Can you work these out from the model? Positions are in its coordinate system, mm. Face numbers are marked on the shaded views. A direction names the side the tool comes from. Coordinates: 2 decimals unless noted, no trailing zeros. Loops run counter-clockwise (first coordinate to the right, second up) from the corner with the lowest first, then second, coordinate; pieces in that order, holes last.
```python
from build123d import *

# Parameters (mm, degrees)
SALIENTE_EXTRUIR1_DEPTH      = 18.75
SALIENTE_EXTRUIR1_DEPTH_BACK = 18.75
CROQUIS1_R                   = 2.45
CROQUIS3_R                   = 1
CORTAR_EXTRUIR1_DEPTH        = 8


with BuildPart() as part:
    # Croquis1 → Saliente-Extruir1 (new, two sides: drawn at the far end of the back side and taken through both)
    with BuildSketch(Plane.XY.offset(-SALIENTE_EXTRUIR1_DEPTH_BACK)):
        Circle(CROQUIS1_R)
    extrude(amount=SALIENTE_EXTRUIR1_DEPTH + SALIENTE_EXTRUIR1_DEPTH_BACK)

    # Croquis3 → Cortar-Extruir1 (cut)
    with BuildSketch(Plane.XY.offset(18.75)):
        Circle(CROQUIS3_R)
        with BuildLine():
            Line((-1.71464282, 1.75), (1.71464282, 1.75))
            ThreePointArc((1.71464282, 1.75), (0, 2.45), (-1.71464282, 1.75))
        make_face()
        with BuildLine():
            Line((-1.71464282, -1.75), (1.71464282, -1.75))
            ThreePointArc((1.71464282, -1.75), (0, -2.45), (-1.71464282, -1.75))
        make_face()
    cortar_extruir1 = extrude(amount=-CORTAR_EXTRUIR1_DEPTH, mode=Mode.SUBTRACT)

    # Simetría1: Cortar-Extruir1 across plane
    add(cortar_extruir1.mirror(Plane.XY), mode=Mode.SUBTRACT)


solid = part.part
```
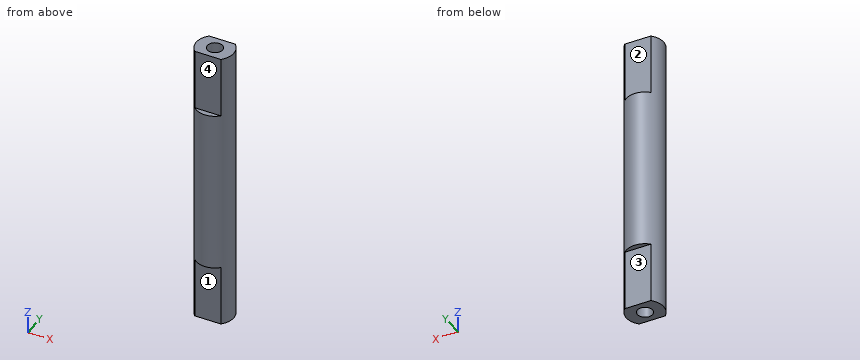
Item 1: On a 3-axis mill with a long thin cutter (end or side, diameter ignored), from which of +Z, -Z, +X, -X, +Y, -Y can I reach the whole of each face in a straight line? I mean the marked faces 1, 2, 3 and 4. Say none if no direction works.
Results are:
face 1: -Z, +X, -X, -Y
face 2: +Z, +X, -X, +Y
face 3: -Z, +X, -X, +Y
face 4: +Z, +X, -X, -Y
Item 2: Suppose I cut it at D-D, the plane z = -2.5. Please give me the cut outline in (x, y), plus the area to 3 significant figures.
Results are:
outline: circle Ø4.9 at (0, 0)
area: 18.9 mm2
Item 3: Suppose I cut it at B-B, the plane x = 0. Please give me the cut outline in (y, z).
Results are:
outline: (-2.45, -10.75) - (-1.75, -10.75) - (-1.75, -18.75) - (-1, -18.75) - (-1, -10.75) - (1, -10.75) - (1, -18.75) - (1.75, -18.75) - (1.75, -10.75) - (2.45, -10.75) - (2.45, 10.75) - (1.75, 10.75) - (1.75, 18.75) - (1, 18.75) - (1, 10.75) - (-1, 10.75) - (-1, 18.75) - (-1.75, 18.75) - (-1.75, 10.75) - (-2.45, 10.75) - close
Item 4: Suppose I cut it at A-A, the plane z = 13.5. Please give me the cut outline in (x, y), plus the area to 3 significant figures.
Results are:
outline: (-1.71, -1.75) - (1.71, -1.75) arc R2.45 ccw to (1.71, 1.75) - (-1.71, 1.75) arc R2.45 ccw to start; hole circle Ø2 at (0, 0)
area: 12.4 mm2
Item 5: Suppose I cut it at C-C, the plane y = -0.6. Please give me the cut outline in (x, z), plus the area to 3 significant figures.
Results are:
outline: (-2.38, -18.75) - (-0.8, -18.75) - (-0.8, -10.75) - (0.8, -10.75) - (0.8, -18.75) - (2.38, -18.75) - (2.38, 18.75) - (0.8, 18.75) - (0.8, 10.75) - (-0.8, 10.75) - (-0.8, 18.75) - (-2.38, 18.75) - close
area: 153 mm2
Item 6: I'm going to push flat-ended pins straight in: P1, Ø1.5, axis at x = 1.5, z = 2, coming from the -Y side; P2, Ø1, axis at x = 0.5, z = -16, coming from the +Y side; P3, Ø1.7, axis at x = -0.5, z = -16, coming from the -Y side. Where does each tip first touch, or does it pass through?
Results are:
P1: stops at y = -2.33
P2: stops at y = 1.75
P3: stops at y = -1.75
Item 7: I need wall thicknesses on line 1 along Y through (x, z) = (0, 15.5); line 2 along Y through (x, z) = (1.2, 11); line 3 along Z through (x, y) = (-0.25, 2.15). Which ranges of each line are inside material? Lowest first, please.
Results are:
line 1: y = -1.75 to -1, 1 to 1.75
line 2: y = -1.75 to 1.75
line 3: z = -10.75 to 10.75
